CAD build for the part. Positions are in the model's coordinates, mm. Give positions to 0.01 mm unless a question says otherwise; leave off trailing zeros. Loops run counter-clockwise (first coordinate to the right, second up) from the corner with the lowest first, then second, coordinate; pieces in that order, holes last.
```python
from build123d import *

# Parameters (mm, degrees)
BOSS_EXTRUDE1_DEPTH = 0.4
SKETCH5_W           = 3
SKETCH5_H           = 0.2
CUT_EXTRUDE1_DEPTH  = 0.7


with BuildPart() as part:
    # Sketch3 → Boss-Extrude1 (new body)
    with BuildSketch(Plane.XY):
        Polygon((0, 0), (0, 2.5), (1.5, 2.5), (1.5, 0.5), (11.5, 0.5), (13, -1), (17.333333334, -1), (18, -1.5), (12, -1.5), (10.5, 0), align=None)
    extrude(amount=BOSS_EXTRUDE1_DEPTH)

    # Sketch5 → Cut-Extrude1 (cut)
    with BuildSketch(Plane(origin=(0, -1, 0), x_dir=(1, 0, 0), z_dir=(0, 1, 0))):
        with Locations((16.5, -0.2)):
            Rectangle(SKETCH5_W, SKETCH5_H)
    extrude(amount=-CUT_EXTRUDE1_DEPTH, mode=Mode.SUBTRACT)


solid = part.part
```
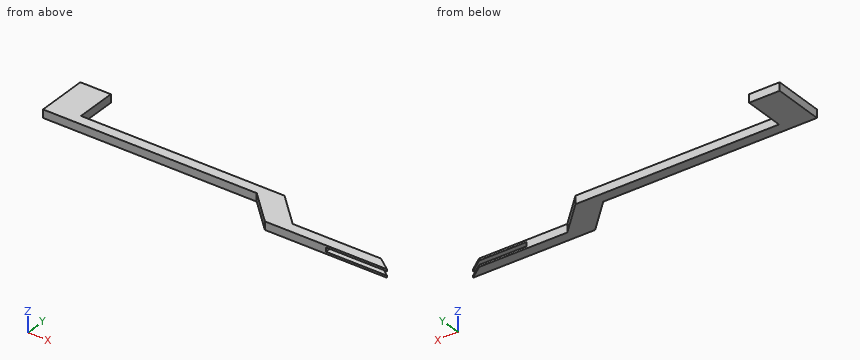
1. Probe line 1 along Y through (x, z) = (10, 0.05); line 2 along Y through (x, z) = (13.75, 0.3); line 3 along X through (y, z) = (1.1, 0.25). List the from-to ranges inside material, lowest first.
Responses:
line 1: y = 0 to 0.5
line 2: y = -1.5 to -1
line 3: x = 0 to 1.5
2. Saw through at C-C, the plane x = 2.5. List the corners of the cut face in (y, z), and give its area (3 significant figures).
Responses:
outline: (0, 0) - (0.5, 0) - (0.5, 0.4) - (0, 0.4) - close
area: 0.200 mm2
3. Saw through at A-A, the plane x = 16.75. List the corners of the cut face in (y, z).
Responses:
outline: (-1.5, 0) - (-1, 0) - (-1, 0.1) - (-1.5, 0.1) - close; (-1.5, 0.3) - (-1, 0.3) - (-1, 0.4) - (-1.5, 0.4) - close
4. Saw through at B-B, the plane y = 0.35. List the corners of the cut face in (x, z).
Responses:
outline: (0, 0) - (11.65, 0) - (11.65, 0.4) - (0, 0.4) - close
